from build123d import *

# Parameters (mm, degrees)
BOSS_EXTRUDE1_DEPTH    = 17
SKETCH10_W             = 3
SKETCH10_H             = 4
SKETCH10_H_2           = 2
BOSS_EXTRUDE8_DEPTH    = 0.4
SKETCH11_W             = 2
SKETCH11_H             = 2.1
SKETCH11_W_2           = 4
BOSS_EXTRUDE9_DEPTH    = 0.4
FILLET5_R              = 0.4
SPLIT2_SURFACE_1_BACK  = 26.421
SPLIT2_SURFACE_1_DEPTH = 52.842
SPLIT2_SURFACE_2_BACK  = 26.421
SPLIT2_SURFACE_2_DEPTH = 52.842
FILLET6_R              = 1.5
SKETCH13_W             = 5.8
SKETCH13_H             = 8.5
BOSS_EXTRUDE10_DEPTH   = 3
FILLET7_R              = 4
SPLIT3_SURFACE_3_BACK  = 34.598
SPLIT3_SURFACE_3_DEPTH = 69.196
SPLIT3_SURFACE_4_BACK  = 34.598
SPLIT3_SURFACE_4_DEPTH = 69.196
CUT_EXTRUDE1_DEPTH     = 1.5
CUT_EXTRUDE2_DEPTH     = 29.664263465


with BuildPart() as part:
    # Sketch1 → Boss-Extrude1 (new body)
    with BuildSketch(Plane.XY):
        Polygon((0, 0), (1.5, 0), (1.5, 10), (13.5, 10), (13.5, 0), (15, 0), (15, 11.5), (0, 11.5), (0, 10), align=None)
    extrude(amount=BOSS_EXTRUDE1_DEPTH)

    # Sketch10 → Boss-Extrude8 (add)
    with BuildSketch(Plane.XZ.offset(-10)):
        with Locations((12, 14)):
            Rectangle(SKETCH10_W, SKETCH10_H)
        with Locations((12, 10)):
            Rectangle(SKETCH10_W, SKETCH10_H_2)
    extrude(amount=BOSS_EXTRUDE8_DEPTH)

    # Sketch11 → Boss-Extrude9 (add)
    with BuildSketch(Plane.ZY.offset(-13.5)):
        with Locations((10, 8.55)):
            Rectangle(SKETCH11_W, SKETCH11_H)
        with Locations((14, 8.55)):
            Rectangle(SKETCH11_W_2, SKETCH11_H)
    extrude(amount=BOSS_EXTRUDE9_DEPTH)

    # Fillet5
    fillet5_edges = [part.edges().sort_by_distance(p)[0] for p in [
        (13.1, 9.6, 10),
        (13.1, 9.6, 14),
    ]]
    fillet(fillet5_edges, radius=FILLET5_R)


with BuildPart() as body_2:
    # Split2: the piece behind the surface
    add(part.part)
    # Split2 surface: a surface, the sketch's curves swept straight by 52.842 mm
    with BuildLine(Plane.XZ.offset(-SPLIT2_SURFACE_1_BACK), mode=Mode.PRIVATE) as split2_surface_1_path:
        Line((15, 8), (0, 8))
    split2_surface_1 = Shell.extrude(split2_surface_1_path.wire(), (0 * SPLIT2_SURFACE_1_DEPTH, -1 * SPLIT2_SURFACE_1_DEPTH, 0 * SPLIT2_SURFACE_1_DEPTH))
    split(bisect_by=split2_surface_1, keep=Keep.BOTTOM)


with BuildPart() as part_1:
    add(part.part)

    # Split2: split by a surface, the side it looks to stays
    # Split2 surface: a surface, the sketch's curves swept straight by 52.842 mm
    with BuildLine(Plane.XZ.offset(-SPLIT2_SURFACE_2_BACK), mode=Mode.PRIVATE) as split2_surface_2_path:
        Line((15, 8), (0, 8))
    split2_surface_2 = Shell.extrude(split2_surface_2_path.wire(), (0 * SPLIT2_SURFACE_2_DEPTH, -1 * SPLIT2_SURFACE_2_DEPTH, 0 * SPLIT2_SURFACE_2_DEPTH))
    split(bisect_by=split2_surface_2, keep=Keep.TOP)

    # Fillet6
    fillet6_edges = [part_1.edges().sort_by_distance(p)[0] for p in [
        (13.5, 10, 4),
        (1.5, 10, 4),
    ]]
    fillet(fillet6_edges, radius=FILLET6_R)


with BuildPart() as body_2_1:
    add(body_2.part)

    # Combine2: union part
    add(part_1.part)

    # Sketch13 → Boss-Extrude10 (add)
    with BuildSketch(Plane.XZ):
        with Locations((-2.9, 4.25)):
            Rectangle(SKETCH13_W, SKETCH13_H)
        with Locations((17.9, 4.25)):
            Rectangle(SKETCH13_W, SKETCH13_H)
    extrude(amount=-BOSS_EXTRUDE10_DEPTH)

    # Fillet7
    fillet7_edges = [body_2_1.edges().sort_by_distance(p)[0] for p in [
        (20.8, 1.5, 8.5),
        (20.8, 1.5, 0),
        (-5.8, 1.5, 0),
        (-5.8, 1.5, 8.5),
    ]]
    fillet(fillet7_edges, radius=FILLET7_R)


with BuildPart() as body_2_2:
    # Split3: the piece behind the surface
    add(body_2_1.part)
    # Split3 surface: a surface, the sketch's curves swept straight by 69.196 mm
    with BuildLine(Plane.ZY.offset(-SPLIT3_SURFACE_3_BACK), mode=Mode.PRIVATE) as split3_surface_3_path:
        Line((0, 3), (17, 3))
    split3_surface_3 = Shell.extrude(split3_surface_3_path.wire(), (-1 * SPLIT3_SURFACE_3_DEPTH, 0 * SPLIT3_SURFACE_3_DEPTH, 0 * SPLIT3_SURFACE_3_DEPTH))
    split(bisect_by=split3_surface_3, keep=Keep.BOTTOM)

    # Sketch16 → Cut-Extrude1 (cut)
    with BuildSketch(Plane(origin=(0, 3, 0), x_dir=(1, 0, 0), z_dir=(0, 1, 0))):
        Polygon((-1, -7.136751346), (1.5, -5.693375673), (1.5, -2.806624327), (-1, -1.363248654), (-3.5, -2.806624327), (-3.5, -5.693375673), align=None)
        Polygon((16, -1.363248654), (13.5, -2.806624327), (13.5, -5.693375673), (16, -7.136751346), (18.5, -5.693375673), (18.5, -2.806624327), align=None)
    extrude(amount=-CUT_EXTRUDE1_DEPTH, mode=Mode.SUBTRACT)

    # Sketch17 → Cut-Extrude2 (cut, through all)
    with BuildSketch(Plane(origin=(0, 1.5, 0), x_dir=(1, 0, 0), z_dir=(0, 1, 0))):
        with BuildLine():
            Line((16, -5.25), (13.5, -5.25))
            Line((13.5, -5.25), (13.5, -3.25))
            Line((13.5, -3.25), (16, -3.25))
            ThreePointArc((16, -3.25), (17, -4.25), (16, -5.25))
        make_face()
        with BuildLine():
            Line((1.5, -3.25), (1.5, -5.25))
            Line((1.5, -5.25), (-1, -5.25))
            ThreePointArc((-1, -5.25), (-2, -4.25), (-1, -3.25))
            Line((-1, -3.25), (1.5, -3.25))
        make_face()
    extrude(amount=-CUT_EXTRUDE2_DEPTH, mode=Mode.SUBTRACT)


with BuildPart() as body_2_3:
    add(body_2_1.part)

    # Split3: split by a surface, the side it looks to stays
    # Split3 surface: a surface, the sketch's curves swept straight by 69.196 mm
    with BuildLine(Plane.ZY.offset(-SPLIT3_SURFACE_4_BACK), mode=Mode.PRIVATE) as split3_surface_4_path:
        Line((0, 3), (17, 3))
    split3_surface_4 = Shell.extrude(split3_surface_4_path.wire(), (-1 * SPLIT3_SURFACE_4_DEPTH, 0 * SPLIT3_SURFACE_4_DEPTH, 0 * SPLIT3_SURFACE_4_DEPTH))
    split(bisect_by=split3_surface_4, keep=Keep.TOP)

    # Combine3: union body 2 2
    add(body_2_2.part)


solid = body_2_3.part
Model file for the job. Use its own axes, mm. A direction names the side the tool comes from. Round coordinates to 2 decimals unless told otherwise and drop trailing zeros. Loops run counter-clockwise (first coordinate to the right, second up) from the corner with the lowest first, then second, coordinate; pieces in that order, holes last. Notation, with made-up numbers: (-19.5, -2.5) - (25.5, -2.5) arc R31 ccw to (25.5, 35.5) - close; hole circle Ø11 at (-31.75, 4). An arc over 180 degrees is marked (long way). Write each question's results on one line, items separated by ' | '.
(1) Mould opens along Z. For faces 1 (the flat face through (1.86, 9.7, 8)), 2 (the flat face through (18.5, 2, 4)), 3 (the flat face through (0, 1, 3.25)), 4 (the flat face through (8, 11.5, 8)) say: released by +Z, released by -Z, zero draft, split by the parting line, or undercut.
Answer below:
face 1: released by +Z | face 2: undercut | face 3: undercut | face 4: zero draft
(2) Wall check: L1, parallel to X at y = 6.75, z = 12.5; L2, parallel to Z at x = 14.75, y = 1; L3, parallel to Y at x = 6.5, z = 8.25. Give the ranges that are in metal, low to high.
Answer below:
L1: x = 0 to 1.5, 13.5 to 15 | L2: z = 0 to 3.25, 5.25 to 17 | L3: y = 10 to 11.5
(3) Saw through at B-B, the plane x = 11.25. List the corners of the cut face in (y, z), then the cut area to 3 significant figures.
Answer below:
outline: (9.6, 9) - (10, 9) - (10, 0) - (11.5, 0) - (11.5, 17) - (10, 17) - (10, 16) - (9.6, 16) - (9.6, 12) - (10, 12) - (10, 11) - (9.6, 11) - close | area: 27.9 mm^2
(4) Saw through at C-C, the plane z = 12.75. List the corners of the cut face in (x, y).
Answer below:
outline: (0, 0) - (1.5, 0) - (1.5, 10) - (10.5, 10) - (10.5, 9.6) - (12.7, 9.6) arc R0.4 cw to (13.1, 9.2) - (13.1, 7.5) - (13.5, 7.5) - (13.5, 0) - (15, 0) - (15, 11.5) - (0, 11.5) - close
(5) 3-axis set-ups, long thin cutter, end or side, ignore diameter. For faces 5 (the flat face through (13.1, 8, 10)), 6 (the flat face through (12.6, 9.8, 9)), 7 (the cylindrical face through (13.07, 9.55, 4.06)), 8 (the flat face through (-2.267, 2.26, 6.405)): which of +Z, -Z, +X, -X, +Y, -Y reach the whole face in a straight line?
Answer below:
face 5: +Z, -Z, -Y | face 6: -Y | face 7: -Z, -Y | face 8: +Y
(6) Saw through at D-D, the plane y = 5.5. List the corners of the cut face in (x, z), then the cut area to 3 significant figures.
Answer below:
outline: (0, 0) - (1.5, 0) - (1.5, 17) - (0, 17) - close; (13.5, 0) - (15, 0) - (15, 17) - (13.5, 17) - close | area: 51.0 mm^2
(7) Pin check, flat tips, straight feed: pin 1 (3 mm diameter, centred on x = -2.5, z = 5.5, fed in from +Y); pin 2 (1.1 mm diameter, centred on x = 12, z = 13, fed in from -Y); pin 3 (2 mm diameter, centred on x = 6, z = 12.5, fed in from -Y). Stop position of each tip, or through.
Answer below:
pin 1: stops at y = 3 | pin 2: stops at y = 9.6 | pin 3: stops at y = 10
(8) Saw through at A-A, the plane y = 1. List the corners of the cut face in (x, z), then the cut area to 3 significant figures.
Answer below:
outline: (-5.8, 4) arc R4 ccw to (-1.8, 0) - (1.5, 0) - (1.5, 3.25) - (-1, 3.25) arc R1 cw to (-1, 5.25) - (1.5, 5.25) - (1.5, 17) - (0, 17) - (0, 8.5) - (-1.8, 8.5) arc R4 ccw to (-5.8, 4.5) - close; (13.5, 0) - (16.8, 0) arc R4 ccw to (20.8, 4) - (20.8, 4.5) arc R4 ccw to (16.8, 8.5) - (15, 8.5) - (15, 17) - (13.5, 17) - (13.5, 5.25) - (16, 5.25) arc R1 cw to (16, 3.25) - (13.5, 3.25) - close | area: 123 mm^2
